Autodesk Inventor part; units mm, degrees
ref_plane "YZ Plane" through (0, 0, 0) normal (1, 0, 0) x (0, 1, 0)
ref_plane "XZ Plane" through (0, 0, 0) normal (0, 1, 0) x (-1, 0, 0)
ref_plane "XY Plane" through (0, 0, 0) normal (0, 0, 1) x (1, 0, 0)
sketch "Boceto1" plane through (0, 0, 0) normal (0, 0, 1) x (1, 0, 0)
  line L0 (0, 0) -> (150, 0)
  line L1 (150, 0) -> (150, 100)
  line L2 (150, 100) -> (0, 100)
  line L3 (0, 100) -> (0, 0)
  dimension "d0" = 150
  dimension "d1" = 100
extrude "Extrusión1" add sketch "Boceto1" along normal blind 3
sketch "Boceto2" plane through (0, 0, 3) normal (0, 0, 1) x (1, 0, 0)
  line L0 (150, 0) -> (150, 100) construction
  line L1 (150, 100) -> (0, 100) construction
  line L2 (0, 100) -> (0, 0) construction
  line L3 (0, 0) -> (150, 0) construction
  line L4 (0, 100) -> (0, 0) construction
  line L5 (0, 50) -> (150, 50) construction
  line L6 (150, 0) -> (150, 100) construction
  line L7 (150, 100) -> (0, 100) construction
  line L8 (122.5, 100) -> (122.5, 0) construction
  line L9 (0, 0) -> (150, 0) construction
  line L10 (0, 66.5) -> (150, 66.5) construction
  line L11 (0, 33.5) -> (150, 33.5) construction
  line L12 (106, 100) -> (106, 0) construction
  line L13 (139, 100) -> (139, 0) construction
  circle A0 centre (106, 50) radius 1.1
  circle A1 centre (122.5, 66.5) radius 1.1
  circle A2 centre (139, 50) radius 1.1
  circle A3 centre (122.5, 33.5) radius 1.1
  line L14 (0, 77.8) -> (150, 77.8) construction
  line L15 (35, 100) -> (35, 0) construction
  line L16 (11, 100) -> (11, 0) construction
  line L17 (59, 100) -> (59, 0) construction
  circle A4 centre (11, 77.8) radius 1.1
  circle A5 centre (59, 77.8) radius 1.1
  line L18 (75, 100) -> (75, 0) construction
  dimension "d4" = 33
  dimension "d5" = 16.5
  dimension "d6" = 33
  dimension "d7" = 16.5
  dimension "d8" = 2.2
  dimension "d9" = 2.2
  dimension "d10" = 2.2
  dimension "d11" = 2.2
  dimension "d15" = 48
  dimension "d16" = 24
  dimension "d17" = 47
  dimension "d18" = 27.8
  dimension "d19" = 2.2
  dimension "d20" = 2.2
  dimension "d22" = 128
  dimension "d24" = 64
extrude "Extrusión2" cut sketch "Boceto2" against normal blind 10
fillet "Empalme1" radius 20 4 edges at (150, 0, 1.5) (150, 100, 1.5) (0, 100, 1.5) (0, 0, 1.5)
sketch "Boceto3" plane through (0, 0, 3) normal (0, 0, 1) x (1, 0, 0)
  circle A0 centre (122.5, 33.5) radius 1.1 construction
  circle A1 centre (106, 50) radius 1.1 construction
  circle A2 centre (11, 77.8) radius 1.1 construction
  circle A3 centre (122.5, 66.5) radius 1.1 construction
  circle A4 centre (139, 50) radius 1.1 construction
  circle A5 centre (59, 77.8) radius 1.1 construction
  arc A6 (0, 20) -> (20, 0) centre (20, 20) ccw construction
  line L0 (20, 0) -> (130, 0) construction
  arc A7 (130, 0) -> (150, 20) centre (130, 20) ccw construction
  line L1 (150, 20) -> (150, 80) construction
  arc A8 (150, 80) -> (130, 100) centre (130, 80) ccw construction
  line L2 (130, 100) -> (20, 100) construction
  arc A9 (20, 100) -> (0, 80) centre (20, 80) ccw construction
  line L3 (0, 80) -> (0, 20) construction
  circle A10 centre (122.5, 66.5) radius 1.1 construction
  line L4 (122.5, 66.5) -> (122.5, 33.5) construction
  circle A11 centre (122.5, 50) radius 25
  line L5 (7.5, 82.8) -> (62.5, 82.8)
  line L6 (62.5, 82.8) -> (62.5, 72.8)
  line L7 (62.5, 72.8) -> (7.5, 72.8)
  line L8 (7.5, 72.8) -> (7.5, 82.8)
  circle A12 centre (11, 77.8) radius 1.1 construction
  circle A13 centre (59, 77.8) radius 1.1 construction
  line L9 (11, 77.8) -> (59, 77.8) construction
  point P0 (0, 0)
  point P1 (35, 77.8)
  dimension "d25" = 50
  dimension "d26" = 10
  dimension "d27" = 55
  dimension "d28" = 27.5
  dimension "d29" = 5
extrude "Extrusión3" add sketch "Boceto3" along normal blind 3
fillet "Empalme2" radius 4 4 edges at (62.5, 82.8, 4.5) (7.5, 82.8, 4.5) (62.5, 72.8, 4.5) (7.5, 72.8, 4.5)
fillet "Empalme3" radius 4 9 edges at (8.6716, 73.9716, 3) (7.5, 77.8, 3) (8.6716, 81.6284, 3) (35, 82.8, 3) (61.3284, 81.6284, 3) (62.5, 77.8, 3) (61.3284, 73.9716, 3) (35, 72.8, 3) (97.5, 50, 3)
sketch "Boceto4" plane through (0, 0, 0) normal (0, 0, -1) x (-1, 0, 0)
  arc A0 (-20, 0) -> (0, 20) centre (-20, 20) ccw construction
  line L0 (0, 80) -> (0, 20) construction
  arc A1 (0, 80) -> (-20, 100) centre (-20, 80) ccw construction
  line L1 (-130, 100) -> (-20, 100) construction
  arc A2 (-130, 100) -> (-150, 80) centre (-130, 80) ccw construction
  line L2 (-150, 20) -> (-150, 80) construction
  arc A3 (-150, 20) -> (-130, 0) centre (-130, 20) ccw construction
  line L3 (-20, 0) -> (-130, 0) construction
  circle A4 centre (-122.5, 33.5) radius 1.1 construction
  circle A5 centre (-106, 50) radius 1.1 construction
  circle A6 centre (-11, 77.8) radius 1.1 construction
  circle A7 centre (-122.5, 66.5) radius 1.1 construction
  circle A8 centre (-139, 50) radius 1.1 construction
  circle A9 centre (-59, 77.8) radius 1.1 construction
  circle A10 centre (-122.5, 33.5) radius 1.1
  circle A11 centre (-122.5, 33.5) radius 1.9
  circle A12 centre (-106, 50) radius 1.1
  circle A13 centre (-106, 50) radius 1.9
  circle A14 centre (-139, 50) radius 1.1
  circle A15 centre (-139, 50) radius 1.9
  circle A16 centre (-122.5, 66.5) radius 1.1
  circle A17 centre (-122.5, 66.5) radius 1.9
  circle A18 centre (-11, 77.8) radius 1.1
  circle A19 centre (-11, 77.8) radius 1.9
  circle A20 centre (-59, 77.8) radius 1.1
  circle A21 centre (-59, 77.8) radius 1.9
  point P0 (0, 0)
  dimension "d34" = 3.8
  dimension "d35" = 3.8
  dimension "d36" = 3.8
  dimension "d37" = 3.8
  dimension "d38" = 3.8
  dimension "d39" = 3.8
extrude "Extrusión4" cut sketch "Boceto4" against normal blind 5 contours A10 | A11 | A12 | A13 | A14 | A15 | A16 | A17 | A18 | A19 | A20 | A21
sketch "Boceto5" plane through (122.5, 33.5, 5) normal (0, 0, -1) x (-1, 0, 0)
  circle A0 centre (111.5, 44.3) radius 1.9 construction
  circle A1 centre (0, 0) radius 1.9 construction
  circle A2 centre (16.5, 16.5) radius 1.9 construction
  circle A3 centre (63.5, 44.3) radius 1.9 construction
  circle A4 centre (0, 33) radius 1.9 construction
  circle A5 centre (-16.5, 16.5) radius 1.9 construction
  arc A6 (102.5, -33.5) -> (122.5, -13.5) centre (102.5, -13.5) ccw construction
  line L0 (122.5, 46.5) -> (122.5, -13.5) construction
  arc A7 (122.5, 46.5) -> (102.5, 66.5) centre (102.5, 46.5) ccw construction
  line L1 (-7.5, 66.5) -> (102.5, 66.5) construction
  arc A8 (-7.5, 66.5) -> (-27.5, 46.5) centre (-7.5, 46.5) ccw construction
  line L2 (-27.5, -13.5) -> (-27.5, 46.5) construction
  arc A9 (-27.5, -13.5) -> (-7.5, -33.5) centre (-7.5, -13.5) ccw construction
  line L3 (102.5, -33.5) -> (-7.5, -33.5) construction
  circle A10 centre (0, 0) radius 1.9
  circle A11 centre (0, 0) radius 1.6
  circle A12 centre (16.5, 16.5) radius 1.9
  circle A13 centre (16.5, 16.5) radius 1.6
  circle A14 centre (-16.5, 16.5) radius 1.9
  circle A15 centre (-16.5, 16.5) radius 1.6
  circle A16 centre (0, 33) radius 1.9
  circle A17 centre (0, 33) radius 1.6
  circle A18 centre (63.5, 44.3) radius 1.9
  circle A19 centre (63.5, 44.3) radius 1.6
  circle A20 centre (111.5, 44.3) radius 1.9
  circle A21 centre (111.5, 44.3) radius 1.6
  point P0 (122.5, -33.5)
  dimension "d42" = 3.2
  dimension "d43" = 3.2
  dimension "d44" = 3.2
  dimension "d45" = 3.2
  dimension "d46" = 3.2
  dimension "d47" = 3.2
extrude "Extrusión5" cut sketch "Boceto5" against normal through all contours A11 | A13 | A15 | A17 | A19 | A21
sketch "Boceto6" plane through (0, 0, 3) normal (0, 0, 1) x (1, 0, 0)
  arc A0 (150, 58.7977) -> (150, 41.2023) centre (122.5, 50) ccw construction
  line L0 (150, 58.7977) -> (150, 80) construction
  arc A1 (150, 80) -> (130, 100) centre (130, 80) ccw construction
  line L1 (130, 100) -> (20, 100) construction
  arc A2 (20, 100) -> (0, 80) centre (20, 80) ccw construction
  line L2 (0, 80) -> (0, 20) construction
  arc A3 (0, 20) -> (20, 0) centre (20, 20) ccw construction
  line L3 (20, 0) -> (130, 0) construction
  arc A4 (130, 0) -> (150, 20) centre (130, 20) ccw construction
  line L4 (150, 20) -> (150, 41.2023) construction
  line L5 (11.5, 68.927) -> (58.5, 68.927) construction
  arc A5 (3.627, 76.8) -> (11.5, 68.927) centre (11.5, 76.8) ccw construction
  line L6 (3.627, 78.8) -> (3.627, 76.8) construction
  arc A6 (11.5, 86.673) -> (3.627, 78.8) centre (11.5, 78.8) ccw construction
  line L7 (58.5, 86.673) -> (11.5, 86.673) construction
  arc A7 (66.373, 78.8) -> (58.5, 86.673) centre (58.5, 78.8) ccw construction
  line L8 (66.373, 76.8) -> (66.373, 78.8) construction
  arc A8 (58.5, 68.927) -> (66.373, 76.8) centre (58.5, 76.8) ccw construction
  line L9 (0, 80) -> (0, 20) construction
  line L10 (0, 95) -> (150, 95) construction
  line L11 (150, 58.7977) -> (150, 80) construction
  line L12 (0, 5) -> (150, 5) construction
  line L13 (150, 20) -> (150, 80) construction
  line L14 (130, 100) -> (20, 100) construction
  line L15 (20, 100) -> (20, 0) construction
  line L16 (20, 0) -> (130, 0) construction
  line L17 (130, 100) -> (130, 0) construction
  circle A9 centre (20, 95) radius 1.6
  circle A10 centre (130, 95) radius 1.6
  circle A11 centre (20, 5) radius 1.6
  circle A12 centre (130, 5) radius 1.6
  point P0 (0, 0)
  dimension "d50" = 20
  dimension "d51" = 5
  dimension "d52" = 20
  dimension "d53" = 5
  dimension "d54" = 3.2
  dimension "d55" = 3.2
  dimension "d56" = 3.2
  dimension "d57" = 3.2
extrude "Extrusión6" cut sketch "Boceto6" against normal through all
equation "\"d5\" = 0.5 * d4"
equation "\"d7\" = d5"
equation "\"d16\" = 0.5 * d15"
equation "\"d24\" = 0.5 * d22"
equation "\"d29\" = 0.5 * d26"
properties part number "base_barra_bola"
Could you check a few things on this model? Use its own coordinates, in mm. A direction names the side the tool comes from. Coordinates: 2 decimals unless noted, no trailing zeros. Order: outer loops, then holes, each group sorted by start corner. A loop starts at its lowest first (then second) coordinate and runs counter-clockwise, first axis right, second up.
Q1. Suppose I cut it at B-B on z = 1.5. Give the number of separate pieces and of enclosed holes in the cut face, and give its area (3 significant figures).
Q2. Suppose I cut it at D-D on y = 5. Please give me the cut outline in (x, z), and give its area (3 significant figures).
Q3. Please list where these lines run through material, in increasing order: L1, parallel to Y at x = 20, z = 1.3; L2, parallel to X at y = 95, z = 1; L3, parallel to Y at x = 59, z = 1.9.
Q4. Will these pins go through, and if not, where does the flat tip stop? pin 1 (3.5 mm diameter, centred on x = 59, y = 77.8, fed in from -Z); pin 2 (12 mm diameter, centred on x = 62.5, y = 32, fed in from +Z); pin 3 (4 mm diameter, centred on x = 139, y = 49.5, fed in from -Z).
Q5. Thinking about a two-plate mould opening in Y: for faces 4 (the flat face through (74, 51, 3)), 5 (the cylindrical face through (11.247, 79.684, 2.465)), 6 (the cylindrical face through (6.014, 94.297, 1.521)), which applies, released by +Y, released by -Y, zero draft, split by the parting line, or undercut?
Q6. Suppose I cut it at C-C on x = 44.5. Please give me the cut outline in (y, z), and give its area (3 significant figures).
Q7. Which directions (+Z, -Z, +X, -X, +Y, -Y) give clear straight access to the entire face, cutting with the end or side of a thin tool? Please do faces 1 (the cylindrical face through (35.329, 71.347, 3.815)), 2 (the cylindrical face through (58.14, 79.15, 5.49)), 3 (the cylindrical face through (107.508, 48.844, 2.465)).
Q8. Suppose I cut it at A-A on y = 50. Please give me the cut outline in (x, z).
Answer:
1. separate pieces: 1
1. enclosed holes: 10
1. area: 14,600 mm2
2. outline: (6.77, 0) - (18.4, 0) - (18.4, 3) - (6.77, 3) - close; (21.6, 0) - (128.4, 0) - (128.4, 3) - (21.6, 3) - close; (131.6, 0) - (143.23, 0) - (143.23, 3) - (131.6, 3) - close
2. area: 390 mm2
3. L1: y = 0 to 3.4, 6.6 to 93.4, 96.6 to 100
3. L2: x = 6.77 to 18.4, 21.6 to 128.4, 131.6 to 143.23
3. L3: y = 0 to 75.9, 79.7 to 100
4. pin 1: stops at z = 5
4. pin 2: stops at z = 3
4. pin 3: stops at z = 0
5. face 4: zero draft
5. face 5: undercut
5. face 6: released by +Y
6. outline: (0, 0) - (100, 0) - (100, 3) - (86.67, 3) arc R4 cw to (82.8, 6) - (72.8, 6) arc R4 cw to (68.93, 3) - (0, 3) - close
6. area: 336 mm2
7. face 1: +Z, -X, -Y
7. face 2: +Z, -Z
7. face 3: -Z
8. outline: (0, 0) - (104.1, 0) - (104.1, 5) - (104.4, 5) - (104.4, 6) - (97.5, 6) arc R4 cw to (93.63, 3) - (0, 3) - close; (107.6, 5) - (107.9, 5) - (107.9, 0) - (137.1, 0) - (137.1, 5) - (137.4, 5) - (137.4, 6) - (107.6, 6) - close; (140.6, 5) - (140.9, 5) - (140.9, 0) - (150, 0) - (150, 3.24) arc R4 cw to (147.5, 6) - (140.6, 6) - close
